Work out the finished part from the listing and answer in its coordinate system (mm). A direction names the side the tool comes from. Round coordinates to 2 decimals unless told otherwise and drop trailing zeros. Write each loop counter-clockwise with the first axis right and the second up, starting at its lowest first coordinate (ties: lowest second). Pieces come first, ordered by that corner, then holes. Notation, with made-up numbers: M -4.5,0.25 L 35.5,0.25 A25 ccw 35.5,24.25 Z; hole C 60.25,-21 d7. An arc over 180 degrees is marked long. One line per item, written item: value. Start each with the question number.
Q1. A tool of negligible diameter and unlimited length cuts with its end or side. For faces 1 (the flat face through (34.25, 29.8, -26.14)), 2 (the flat face through (74.708, 0, -13)), 3 (the flat face through (74, 0, -2.5)), from which of +Z, -Z, +X, -X, +Y, -Y can it reach the whole face along a straight path? Write none if from no direction.
Q2. Consider probe 1 along Y at (x, z) = (40, -5); probe 2 along Z at (x, y) = (39, -15); probe 3 along X at (y, z) = (25.5, -4.5). Determine where each line is inside the solid, lowest interval first.
Q3. Given pin 1 Ø1 at (x, y) = (74, 1.5) entering from -Z; pin 2 Ø1.5 at (y, z) = (-8, -16) entering from -X, each flat-ended and moving along its own axis, determine where each tip first touches the part or whether it passes through.
Q4. Find section C-C (y = -20). Write down the section's boundary in (x, z).
Q5. The mould has two halves that part along Y. Classify faces 4 (the flat face through (39, -33, -14)), 5 (the flat face through (0, 0, -7)), 6 (the flat face through (38, 35, -15)): released by +Y, released by -Y, zero draft, split by the parting line, or undercut.
Q6. Find section B-B (x = 47). Write down the section's boundary in (y, z).
Q7. Find section D-D (z = -22.5). Write down the section's boundary in (x, y), and give its area (3 significant figures).
Q8. Find section A-A (y = -1.5). Write down the section's boundary in (x, z), and give its area (3 significant figures).
from build123d import *

# Parameters (mm, degrees)
BOSS_EXTRUDE1_DEPTH      = 35
BOSS_EXTRUDE1_DEPTH_BACK = 35
CUT_EXTRUDE1_DEPTH       = 33
CUT_EXTRUDE1_DEPTH_BACK  = 33
CUT_EXTRUDE2_REACH       = 92.823
SKETCH3_W                = 10
SKETCH3_H                = 20
BOSS_EXTRUDE8_DEPTH      = 20
SKETCH5_R                = 1.5
CUT_EXTRUDE3_DEPTH       = 19.999999693


with BuildPart() as part:
    # Sketch1 → Boss-Extrude1 (new, two sides: drawn at the far end of the back side and taken through both)
    with BuildSketch(Plane(origin=(0, 0, 0), x_dir=(1, 0, 0), z_dir=(0, 1, 0)).offset(-BOSS_EXTRUDE1_DEPTH_BACK)):
        Polygon((0, 15), (19.283628291, 37.981333294), (74.707976009, 15), (74.707976009, 0), (0, 0), align=None)
    extrude(amount=BOSS_EXTRUDE1_DEPTH + BOSS_EXTRUDE1_DEPTH_BACK)

    # Sketch2 → Cut-Extrude1 (cut, two sides: drawn at the far end of the back side and taken through both)
    with BuildSketch(Plane(origin=(0, 0, 0), x_dir=(1, 0, 0), z_dir=(0, 1, 0)).offset(-CUT_EXTRUDE1_DEPTH_BACK)):
        Polygon((21.032566766, 35.091034272), (72.707976009, 13.664173121), (72.707976009, 2), (36.573879749, 2), (1.347807304, 16.606254197), (17.935820986, 36.375079097), align=None)
    extrude(amount=CUT_EXTRUDE1_DEPTH + CUT_EXTRUDE1_DEPTH_BACK, mode=Mode.SUBTRACT)

    # Sketch3 → Cut-Extrude2 (cut, up to next)
    with BuildSketch(Plane(origin=(74.707976009, 0, 0), x_dir=(0, 0, -1), z_dir=(1, 0, 0)), mode=Mode.PRIVATE) as cut_extrude2_sk1:
        with Locations((7.5, 0)):
            Rectangle(SKETCH3_W, SKETCH3_H)
    cut_extrude2_tool1 = extrude(cut_extrude2_sk1.sketch, amount=-CUT_EXTRUDE2_REACH, mode=Mode.PRIVATE) & part.part
    add(cut_extrude2_tool1.solids().sort_by_distance((74.707976, 0, -7.5))[0], mode=Mode.SUBTRACT)

    # 3DSketch2 → Boss-Extrude8 (add, along a direction that is not the sketch's normal)
    with BuildSketch(Plane(origin=(17.935820986, -33, -36.375079097), x_dir=(-0.23407626920535343, 0.9313371729360082, 0.2789612347665302), z_dir=(-0.7660444431189789, 0, -0.6427876096865383))):
        with BuildLine():
            Line((0, 0), (2.184948176, -5.588023038))
            ThreePointArc((2.184948176, -5.588023038), (5.496320655, -2.406337312), (5.588023038, 2.184948176))
            Line((5.588023038, 2.184948176), (0, 0))
        make_face()
        with BuildLine():
            Line((61.468253414, 24.034429934), (55.880230376, 21.849481758))
            ThreePointArc((55.880230376, 21.849481758), (59.061916102, 18.538109279), (63.65320159, 18.446406897))
            Line((63.65320159, 18.446406897), (61.468253414, 24.034429934))
        make_face()
        with BuildLine():
            Line((70.865849574, 0), (68.680901398, 5.588023038))
            ThreePointArc((68.680901398, 5.588023038), (65.369528919, 2.406337312), (65.277826536, -2.184948176))
            Line((65.277826536, -2.184948176), (70.865849574, 0))
        make_face()
        with BuildLine():
            Line((9.39759616, -24.034429934), (14.985619198, -21.849481758))
            ThreePointArc((14.985619198, -21.849481758), (11.803933472, -18.538109279), (7.212647984, -18.446406897))
            Line((7.212647984, -18.446406897), (9.39759616, -24.034429934))
        make_face()
    extrude(amount=-BOSS_EXTRUDE8_DEPTH, dir=(-0.9237391286459794, 0, -0.38302222155948973))

    # Sketch5 → Cut-Extrude3 (cut, along a direction that is not the sketch's normal)
    with BuildSketch(Plane(origin=(-7.386058148, 0, -6.197638667), x_dir=(-0.6427876096865378, 0, 0.7660444431189795), z_dir=(-0.7660444431189795, 0, -0.6427876096865378))):
        with Locations((-37.490666647, -31)):
            Circle(SKETCH5_R)
        with Locations((-37.490666647, 31)):
            Circle(SKETCH5_R)
        with Locations((-15.490666647, 31)):
            Circle(SKETCH5_R)
        with Locations((-15.490666647, -31)):
            Circle(SKETCH5_R)
    extrude(amount=-CUT_EXTRUDE3_DEPTH, dir=(-0.9237391286459794, 0, -0.38302222155948973), mode=Mode.SUBTRACT)


solid = part.part
The answers:
1. face 1: none
1. face 2: +Z, -Z, +X, +Y, -Y
1. face 3: +X
2. probe 1: -35 to -33, 33 to 35
2. probe 2: -29.81 to -27.64, -2 to 0
2. probe 3: 0 to 30.54, 72.71 to 74.71
3. pin 1: z = -15.5
3. pin 2: x = 0.21
4. outline: M 0,-15 L 1.35,-16.61 L 36.57,-2 L 72.71,-2 L 72.71,-13.66 L 17.94,-36.38 L 19.28,-37.98 L 74.71,-15 L 74.71,0 L 0,0 Z
5. face 4: undercut
5. face 5: zero draft
5. face 6: released by +Y
6. outline: M -35,-26.49 L 35,-26.49 L 35,0 L -35,0 Z; hole M -33,-24.32 L 33,-24.32 L 33,-2 L -33,-2 Z
7. outline: M 6.29,-35 L 56.62,-35 L 56.62,35 L 6.29,35 L 6.29,33 L 51.4,33 L 51.4,-33 L 6.29,-33 Z
7. area: 546 mm2
8. outline: M 0,-15 L 1.35,-16.61 L 36.57,-2 L 72.71,-2 L 72.71,-2.5 L 74.71,-2.5 L 74.71,0 L 0,0 Z; M 17.94,-36.38 L 19.28,-37.98 L 74.71,-15 L 74.71,-12.5 L 72.71,-12.5 L 72.71,-13.66 Z
8. area: 549 mm2
